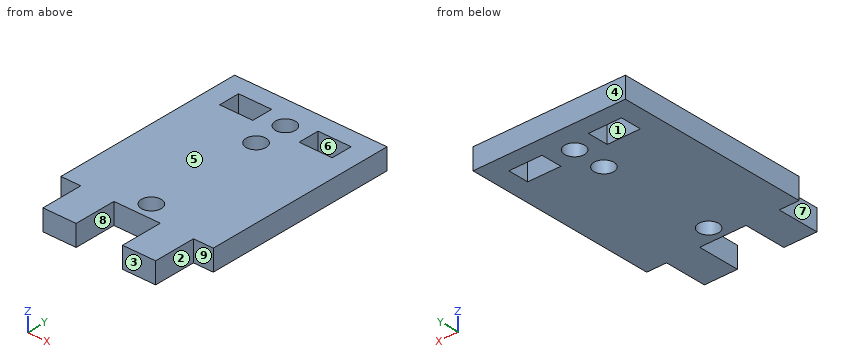
```python
from build123d import *

# Parameters (mm, degrees)
BOSS_EXTRUDE1_DEPTH = 3.175
SKETCH2_R           = 1.5
CUT_EXTRUDE1_DEPTH  = 22.594689741
SKETCH3_R           = 1.5
SKETCH3_W           = 5
SKETCH3_H           = 3.175
CUT_EXTRUDE2_DEPTH  = 22.594689741


with BuildPart() as part:
    # Sketch1 → Boss-Extrude1 (new body)
    with BuildSketch(Plane.XY):
        Polygon((-11.5, 0), (-11.5, -11.2), (-8.5, -11.2), (-8.5, -17.55), (-3.5, -17.55), (-3.5, -11.2), (3.5, -11.2), (3.5, -17.55), (8.5, -17.55), (8.5, -11.2), (11.5, -11.2), (11.5, 0), (11.5, 18), (-11.5, 18), align=None)
    extrude(amount=BOSS_EXTRUDE1_DEPTH)

    # Sketch2 → Cut-Extrude1 (cut, through all)
    with BuildSketch(Plane.XY.offset(3.175)):
        with Locations((0, -8.8)):
            Circle(SKETCH2_R)
        with Locations(Location((0, 8.8, 0), (0, 0, 180))):
            Circle(SKETCH2_R)
    extrude(amount=-CUT_EXTRUDE1_DEPTH, mode=Mode.SUBTRACT)

    # Sketch3 → Cut-Extrude2 (cut, through all)
    with BuildSketch(Plane.XY.offset(3.175)):
        with Locations((0, 13.72908257)):
            Circle(SKETCH3_R)
        with Locations((6, 13.72908257)):
            Rectangle(SKETCH3_W, SKETCH3_H)
        with Locations((-6, 13.72908257)):
            Rectangle(SKETCH3_W, SKETCH3_H)
    extrude(amount=-CUT_EXTRUDE2_DEPTH, mode=Mode.SUBTRACT)


solid = part.part
```
Part model, mm, in its own coordinate system. Face numbers are marked on the shaded views. A direction names the side the tool comes from. Coordinates: 2 decimals unless noted, no trailing zeros. Loops run counter-clockwise (first coordinate to the right, second up) from the corner with the lowest first, then second, coordinate; pieces in that order, holes last. Notation, with made-up numbers: (-5.75, -39.75) - (31.25, -39.75) arc R10 cw to (31.25, -30.75) - close; hole circle Ø3 at (-31, 0). An arc over 180 degrees is marked (long way). Write item = value, one per line. Start each with the question number.
Item 1: Cut at C-C, the plane x = 0. Give the cut face in (y, z) (3 decimals), and give its area (3 significant figures).
Item 2: 3-axis set-ups, long thin cutter, end or side, ignore diameter. For the marked faces 5, 6, 7, 8 and 9: which of +Z, -Z, +X, -X, +Y, -Y reach the whole face in a straight line?
Item 3: Wall check: L1, parallel to Y at x = 0, z = 1.4; L2, parallel to Y at x = -7.25, z = 2.6; L3, parallel to X at y = 13.5, z = 2.45. Give the ranges that are in metal, low to high. Write a range as from..to.
Item 4: Flat gauge pins, fed straight in: pin 1 Ø1 at (x, y) = (8, -12.5) entering from -Z; pin 2 Ø1.6 at (y, z) = (-15, 1) entering from +X; pin 3 Ø1.5 at (x, z) = (-10.5, 2) entering from -Y; pin 4 Ø1 at (y, z) = (-13, 2) entering from -X. Where does each tip first touch, or does it go through?
Item 5: Cut at B-B, the plane y = -8.8. Give the cut face in (x, z) (3 decimals).
Item 6: Cut at D-D, the plane z = 1.4. Give the cut face in (x, y).
Item 7: Mould opens along Y. For the marked faces 1, 2, 3 and 4 say: released by +Y, released by -Y, zero draft, split by the parting line, or undercut.
Item 8: Cut at A-A, the plane x = 5. Give the cut face in (y, z) (3 decimals).
The answers:
q1.outline = (-11.2, 0) - (-10.3, 0) - (-10.3, 3.175) - (-11.2, 3.175) - close; (-7.3, 0) - (7.3, 0) - (7.3, 3.175) - (-7.3, 3.175) - close; (10.3, 0) - (12.229, 0) - (12.229, 3.175) - (10.3, 3.175) - close; (15.229, 0) - (18, 0) - (18, 3.175) - (15.229, 3.175) - close
q1.area = 64.1 mm2
q2.face_5 = +Z, +X, -X, +Y, -Y
q2.face_6 = +Z, -Z
q2.face_7 = +Z, -Z, -X, -Y
q2.face_8 = +Z, -Z, -Y
q2.face_9 = +Z, -Z, +X, -Y
q3.L1 = -11.2..-10.3, -7.3..7.3, 10.3..12.23, 15.23..18
q3.L2 = -17.55..12.14, 15.32..18
q3.L3 = -11.5..-8.5, -3.5..-1.48, 1.48..3.5, 8.5..11.5
q4.pin_1 = 0
q4.pin_2 = 8.5
q4.pin_3 = -11.2
q4.pin_4 = -8.5
q5.outline = (-11.5, 0) - (-1.5, 0) - (-1.5, 3.175) - (-11.5, 3.175) - close; (1.5, 0) - (11.5, 0) - (11.5, 3.175) - (1.5, 3.175) - close
q6.outline = (-11.5, -11.2) - (-8.5, -11.2) - (-8.5, -17.55) - (-3.5, -17.55) - (-3.5, -11.2) - (3.5, -11.2) - (3.5, -17.55) - (8.5, -17.55) - (8.5, -11.2) - (11.5, -11.2) - (11.5, 18) - (-11.5, 18) - close; hole (-8.5, 12.14) - (-3.5, 12.14) - (-3.5, 15.32) - (-8.5, 15.32) - close; hole circle Ø3 at (0, -8.8); hole circle Ø3 at (0, 8.8); hole circle Ø3 at (0, 13.73); hole (3.5, 12.14) - (8.5, 12.14) - (8.5, 15.32) - (3.5, 15.32) - close
q7.face_1 = undercut
q7.face_2 = zero draft
q7.face_3 = released by -Y
q7.face_4 = released by +Y
q8.outline = (-17.55, 0) - (12.142, 0) - (12.142, 3.175) - (-17.55, 3.175) - close; (15.317, 0) - (18, 0) - (18, 3.175) - (15.317, 3.175) - close
